Design review of the part built by this model. Coordinates are the model's own, in mm. A direction names the side the tool comes from. Coordinates: 2 decimals unless noted, no trailing zeros. Order: outer loops, then holes, each group sorted by start corner. A loop starts at its lowest first (then second) coordinate and runs counter-clockwise, first axis right, second up. Notation, with made-up numbers: (62.25, -20) -> (116.25, -20) arc R18 cw to (116.25, 3) -> close; hole circle Ø6 at (11, 78.25). An arc over 180 degrees is marked (long way). Write item = value, one per line.
```python
from build123d import *

# Parameters (mm, degrees)
SKETCH_1_W      = 25
SKETCH_1_H      = 30
SKETCH_1_R      = 1.7
EXTRUDE_1_DEPTH = 4
SKETCH_2_W      = 25
SKETCH_2_H      = 4
EXTRUDE_2_DEPTH = 50
EXTRUDE_3_DEPTH = 25
SKETCH_4_R      = 2.9
EXTRUDE_4_DEPTH = 5
CHAMFER_2_SIZE  = 5


with BuildPart() as part:
    # 草图1 → 凸台-拉伸1 (new body)
    with BuildSketch(Plane(origin=(0, 0, 0), x_dir=(1, 0, 0), z_dir=(0, 1, 0))):
        with Locations((12.5, 15)):
            Rectangle(SKETCH_1_W, SKETCH_1_H)
        with Locations(Location((5, 22.5, 0), (0, 0, 270))):
            Circle(SKETCH_1_R, mode=Mode.SUBTRACT)
        with Locations(Location((20, 22.5, 0), (0, 0, 270))):
            Circle(SKETCH_1_R, mode=Mode.SUBTRACT)
    extrude(amount=EXTRUDE_1_DEPTH)

    # 草图2 → 凸台-拉伸2 (add)
    with BuildSketch(Plane(origin=(0, 4, 0), x_dir=(1, 0, 0), z_dir=(0, 1, 0))):
        with Locations((12.5, 2)):
            Rectangle(SKETCH_2_W, SKETCH_2_H)
    extrude(amount=EXTRUDE_2_DEPTH)

    # 草图3 → 凸台-拉伸3 (add)
    with BuildSketch(Plane(origin=(25, 0, 0), x_dir=(0, 0, -1), z_dir=(1, 0, 0))):
        Polygon((4, 4), (4, 9), (9, 4), align=None)
    extrude(amount=-EXTRUDE_3_DEPTH)

    # 草图4 → 凸台-拉伸4 (add)
    with BuildSketch(Plane(origin=(0, 0, -4), x_dir=(-1, 0, 0), z_dir=(0, 0, -1))):
        with Locations(Location((-12.5, 39, 0), (0, 0, 180))):
            Circle(SKETCH_4_R)
    extrude(amount=EXTRUDE_4_DEPTH)

    # 倒角2
    chamfer_2_edges = [part.edges().sort_by_distance(p)[0] for p in [
        (0, 54, -2),
        (25, 54, -2),
    ]]
    chamfer(chamfer_2_edges, length=CHAMFER_2_SIZE)


solid = part.part
```
(1) We need section C-C (x = 12.5). Write out the cut boundary in (y, z), and give its area (4 significant figures).
Report:
outline = (0, -30) -> (4, -30) -> (4, -9) -> (9, -4) -> (36.1, -4) -> (36.1, -9) -> (41.9, -9) -> (41.9, -4) -> (54, -4) -> (54, 0) -> (0, 0) -> close
area = 361.5 mm²
(2) We need section D-D (z = -26.25). Write out the cut boundary in (x, y).
Report:
outline = (0, 0) -> (25, 0) -> (25, 4) -> (0, 4) -> close
(3) Insertion check: pin 1 (1.7 mm diameter, centred on x = 13, y = 39.5, fed in from -Z); pin 2 (6.5 mm diameter, centred on x = 15.5, z = -19, fed in from +Y); pin 3 (8 mm diameter, centred on x = 13, y = 12.5, fed in from -Z). Each pin has a flat end and moves straight along its axis. Give the tip position at first contact, or say it passes through.
Report:
pin_1 = -9
pin_2 = 4
pin_3 = -4.5
(4) For L1, parallel to X at y = 1.9, z = -22.5; L2, parallel to Z at x = 19.75, y = 17; L3, parallel to Y at x = 8.75, z = -17.25, list the stretches that pass through material, from the lowest coordinate up.
Report:
L1 = 0 to 3.3, 6.7 to 18.3, 21.7 to 25
L2 = -4 to 0
L3 = 0 to 4
(5) For faces 1 (the flat face through (3, 52, -2)), 2 (the flat face through (12, 4, -20)), 3 (the cylindrical face through (10.199, 40.765, -6.465)), list the 3-axis set-ups (+Z, -Z, +X, -X, +Y, -Y) from which the entire face can be reached by the end or side of a thin tool; tool diameter is ignored.
Report:
face_1 = +Z, -Z, -X, +Y
face_2 = -Z, +X, -X, +Y
face_3 = -Z
(6) The part is to be moulded in two halves that separate along Y. For faces 4 (the flat face through (12, 39, -9)), 5 (the flat face through (13, 7, -6)), 6 (the flat face through (12, 0, -15)), say which applies: released by +Y, released by -Y, zero draft, split by the parting line, or undercut.
Report:
face_4 = zero draft
face_5 = undercut
face_6 = released by -Y
(7) We need section B-B (y = 39). Write out the cut boundary in (x, z), and give its area (3 significant figures).
Report:
outline = (0, -4) -> (9.6, -4) -> (9.6, -9) -> (15.4, -9) -> (15.4, -4) -> (25, -4) -> (25, 0) -> (0, 0) -> close
area = 129 mm²
(8) We need section A-A (z = -22.5). Write out the cut boundary in (x, y), and give its area (3 significant figures).
Report:
outline = (0, 0) -> (3.3, 0) -> (3.3, 4) -> (0, 4) -> close; (6.7, 0) -> (18.3, 0) -> (18.3, 4) -> (6.7, 4) -> close; (21.7, 0) -> (25, 0) -> (25, 4) -> (21.7, 4) -> close
area = 72.8 mm²
